from build123d import *

# Parameters (mm, degrees)
BOSS_EXTRUDE1_DEPTH     = 19
BOSS_EXTRUDE2_START     = -5
BOSS_EXTRUDE2_DEPTH     = 5
CUT_EXTRUDE1_DEPTH      = 295.487690744
CUT_EXTRUDE1_DEPTH_BACK = 295.487690744
SKETCH3_R               = 1.5
SKETCH4_R               = 29
BOSS_EXTRUDE3_DEPTH     = 3
SKETCH5_R               = 18.5
CUT_EXTRUDE2_DEPTH      = 4
CUT_EXTRUDE3_DEPTH      = 295.553899991
CUT_EXTRUDE3_DEPTH_BACK = 295.553899991
SKETCH6_R               = 15.5
FILLET1_R               = 10
CUT_EXTRUDE4_DEPTH      = 295.487690751
CUT_EXTRUDE4_DEPTH_BACK = 295.487690751
SKETCH7_R               = 10


with BuildPart() as part:
    # Sketch1 → Boss-Extrude1 (new body)
    with BuildSketch(Plane(origin=(0, 0, 0), x_dir=(1, 0, 0), z_dir=(0, 1, 0))):
        with BuildLine():
            Line((0, -41), (250, -41))
            ThreePointArc((250, -41), (291, 0), (250, 41))
            Line((250, 41), (0, 41))
            ThreePointArc((0, 41), (-41, 0), (0, -41))
        make_face()
        with BuildLine():
            Line((0, 29), (250, 29))
            ThreePointArc((250, 29), (279, 0), (250, -29))
            Line((250, -29), (0, -29))
            ThreePointArc((0, -29), (-29, 0), (0, 29))
        make_face(mode=Mode.SUBTRACT)
    extrude(amount=BOSS_EXTRUDE1_DEPTH)

    # Sketch1<2> → Boss-Extrude2 (add)
    with BuildSketch(Plane(origin=(0, 0, 0), x_dir=(1, 0, 0), z_dir=(0, 1, 0)).offset(BOSS_EXTRUDE2_START)):
        with BuildLine():
            ThreePointArc((0, 41), (-41, 0), (0, -41))
            Line((0, -41), (250, -41))
            ThreePointArc((250, -41), (291, 0), (250, 41))
            Line((250, 41), (0, 41))
        make_face()
    extrude(amount=BOSS_EXTRUDE2_DEPTH)

    # Sketch3 → Cut-Extrude1 (cut, two sides: drawn at the far end of the back side and taken through both)
    with BuildSketch(Plane(origin=(0, 0, 0), x_dir=(1, 0, 0), z_dir=(0, 1, 0)).offset(-CUT_EXTRUDE1_DEPTH_BACK)):
        with Locations(Location((0, 15, 0), (0, 0, 270))):
            Circle(SKETCH3_R)
        with Locations(Location((15, 0, 0), (0, 0, 270))):
            Circle(SKETCH3_R)
        with Locations(Location((0, -15, 0), (0, 0, 270))):
            Circle(SKETCH3_R)
        with Locations(Location((-15, 0, 0), (0, 0, 270))):
            Circle(SKETCH3_R)
    extrude(amount=CUT_EXTRUDE1_DEPTH + CUT_EXTRUDE1_DEPTH_BACK, mode=Mode.SUBTRACT)

    # Sketch4 → Boss-Extrude3 (add)
    with BuildSketch(Plane(origin=(0, 0, 0), x_dir=(1, 0, 0), z_dir=(0, 1, 0))):
        with Locations((250, 0)):
            Circle(SKETCH4_R)
    extrude(amount=BOSS_EXTRUDE3_DEPTH)

    # Sketch5 → Cut-Extrude2 (cut)
    with BuildSketch(Plane(origin=(0, 3, 0), x_dir=(1, 0, 0), z_dir=(0, 1, 0))):
        with Locations(Location((250, 0, 0), (0, 0, 270))):
            Circle(SKETCH5_R)
    extrude(amount=-CUT_EXTRUDE2_DEPTH, mode=Mode.SUBTRACT)

    # Sketch6 → Cut-Extrude3 (cut, two sides: drawn at the far end of the back side and taken through both)
    with BuildSketch(Plane(origin=(0, -1, 0), x_dir=(1, 0, 0), z_dir=(0, 1, 0)).offset(-CUT_EXTRUDE3_DEPTH_BACK)):
        with Locations(Location((250, 0, 0), (0, 0, 270))):
            Circle(SKETCH6_R)
    extrude(amount=CUT_EXTRUDE3_DEPTH + CUT_EXTRUDE3_DEPTH_BACK, mode=Mode.SUBTRACT)

    # Fillet1
    # the kernel refuses this fillet: 10 mm, written as the material it adds along each edge
    with BuildSketch(Plane(origin=(250, 0, 0), x_dir=(0.5782894613752282, 0, -0.8158316608604672), z_dir=(0.8158316608604672, 0, 0.5782894613752282))) as fillet1_piece_1:
        with BuildLine():
            CenterArc((36.141428429, 10), FILLET1_R, 224.427004001, 45.572995999)
            Line((36.141428429, 0), (36.141428429, -0.2))
            Line((36.141428429, -0.2), (29, -0.2))
            Line((29, -0.2), (28.8, 0))
            ThreePointArc((28.8, 0), (28.8, 1.5), (28.857171431, 2.86))
            Line((28.857171431, 2.86), (29, 3))
        make_face()
    revolve(axis=Axis((250, 0, 0), (0, 1, 0)), revolution_arc=250.660644369)

    # Sketch7 → Cut-Extrude4 (cut, two sides: drawn at the far end of the back side and taken through both)
    with BuildSketch(Plane(origin=(0, 0, 0), x_dir=(1, 0, 0), z_dir=(0, 1, 0)).offset(-CUT_EXTRUDE4_DEPTH_BACK)):
        with Locations(Location((70.3, 0, 0), (0, 0, 270))):
            Circle(SKETCH7_R)
    extrude(amount=CUT_EXTRUDE4_DEPTH + CUT_EXTRUDE4_DEPTH_BACK, mode=Mode.SUBTRACT)


solid = part.part
For this review, take the finished solid that the model builds, in its own axes (mm). A direction names the side the tool comes from. Give positions to 0.01 mm unless a question says otherwise; leave off trailing zeros. Order: outer loops, then holes, each group sorted by start corner. A loop starts at its lowest first (then second) coordinate and runs counter-clockwise, first axis right, second up. Notation, with made-up numbers: (-26.5, -27) - (5.5, -27) arc R34 cw to (5.5, 12) - close; hole circle Ø11 at (81.25, 9). An arc over 180 degrees is marked (long way). Answer as a JSON object with one key per item and string values. Group by question number.
Item 1: Wall thickness on line 1 along X through (y, z) = (-2.95, 0); line 2 along Z through (x, y) = (250, -4.15); line 3 along Z through (x, y) = (37.5, 0.25): over which ranges is each line inside the solid? List them lowest first.
Item 2: Take a section at B-B on x = 70.3. Give the boundary of the cut face in (y, z).
Item 3: Machinability: for faces 1 (the flat face through (269, 3, 0)), 2 (the flat face through (123, -5, -1)), which of the approach directions +Z, -Z, +X, -X, +Y, -Y give a long, thin tool a straight path to every point of the face, cutting with its end or side? Answer none if there is none.
Item 4: Draft analysis for pull direction X (two halves, no side actions). For faces 3 (the flat face through (127, 7, -41)), 4 (the cylindrical face through (-40.99, 6.83, -0.9)), 5 (the cylindrical face through (278.993, 10.888, -0.638)), state which applies: pulls with the +X half, pulls with the -X half, needs draft (parallel to the pull), parting line crosses it, or undercut.
Item 5: Clearance check with flat-ended pins moving along their axes: pin 1 Ø3.5 at (x, z) = (15, 0) entering from +Y; pin 2 Ø1.8 at (x, z) = (-15, 0) entering from +Y; pin 3 Ø1 at (y, z) = (5.5, -31.5) entering from +X; pin 4 Ø8 at (y, z) = (7.5, -19) entering from +X. State where each tip first meets the part, or that it passes through.
Item 6: Take a section at C-C on x = 173. Give the boundary of the cut face in (y, z).
Item 7: Take a section at A-A on y = 8. Give the boundary of the cut face in (x, z), and give its area (3 significant figures).
Reported:
{
 "1": {"line 1": "-41 to -16.5, -13.5 to 13.5, 16.5 to 60.3, 80.3 to 234.5, 265.5 to 291", "line 2": "-41 to -15.5, 15.5 to 41", "line 3": "-41 to -29, 29 to 41"},
 "2": {"outline": "(-5, -41) - (19, -41) - (19, -29) - (0, -29) - (0, -10) - (-5, -10) - close; (-5, 10) - (0, 10) - (0, 29) - (19, 29) - (19, 41) - (-5, 41) - close"},
 "3": {"face 1": "+Y", "face 2": "+Z, -Z, +X, -X, -Y"},
 "4": {"face 3": "needs draft", "face 4": "pulls with the -X half", "face 5": "undercut"},
 "5": {"pin 1": "y = 0", "pin 2": "through", "pin 3": "x = 276.83", "pin 4": "x = 288.16"},
 "6": {"outline": "(-5, -41) - (19, -41) - (19, -29) - (0, -29) - (0, 29) - (19, 29) - (19, 41) - (-5, 41) - close"},
 "7": {"outline": "(0, -41) - (250, -41) arc R41 ccw to (250, 41) - (0, 41) arc R41 ccw to start; hole (0, -29) - (250, -29) arc R29 ccw to (250, 29) - (0, 29) arc R29 ccw to start", "area": "8,640 mm^2"}
}
